Check sheet for the modelled part. Datum: model origin and axes. Units: mm. Face numbers are marked on the shaded views. A direction names the side the tool comes from. Coordinates: 2 decimals unless noted, no trailing zeros. Loops run counter-clockwise (first coordinate to the right, second up) from the corner with the lowest first, then second, coordinate; pieces in that order, holes last.
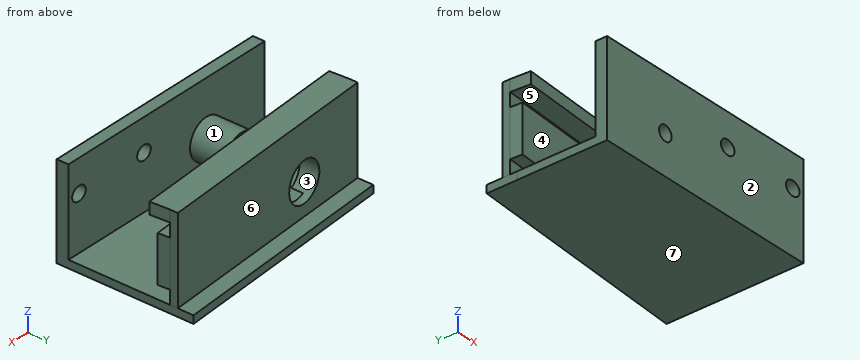
Autodesk Inventor part; units mm, degrees
ref_plane "YZ Plane" through (0, 0, 0) normal (1, 0, 0) x (0, 1, 0)
ref_plane "XZ Plane" through (0, 0, 0) normal (0, 1, 0) x (-1, 0, 0)
ref_plane "XY Plane" through (0, 0, 0) normal (0, 0, 1) x (1, 0, 0)
ref_plane "작업 평면1" through (-108.7402, -145.9081, -64.7043) normal (0, -1, 0) x (1, 0, 0)
sketch "스케치1" plane through (-108.7402, -145.9081, -64.7043) normal (0, -1, 0) x (1, 0, 0)
  ellipse E0 centre (-21.9712, -11.93) end of major axis (-19.8923, -11.93) minor radius 1.7957
  ellipse E1 centre (-2.1698, -11.93) end of major axis (-0.091, -11.93) minor radius 1.7957
  line L0 (-25.1804, -13.5798) -> (-25.1804, 0)
  ellipse E2 centre (0, 0) end of major axis (1.0394, 0) minor radius 0.8978 (1.0394, 0) -> (0, 0.8978) ccw
  line L1 (1.0394, 0) -> (1.0394, -13.5798)
  ellipse E3 centre (-0.2599, -13.5798) end of major axis (1.0394, -13.5798) minor radius 1.1223 (-0.2599, -14.7021) -> (1.0394, -13.5798) ccw
  line L2 (-0.2599, -14.7021) -> (-23.8811, -14.7021)
  ellipse E4 centre (-23.8811, -13.5798) end of major axis (-22.5818, -13.5798) minor radius 1.1223 (-25.1804, -13.5798) -> (-23.8811, -14.7021) ccw
  line L3 (-25.1804, -13.5798) -> (-25.1804, 0)
  ellipse E5 centre (-24.141, 0) end of major axis (-25.1804, 0) minor radius 0.8978 (-24.141, 0.8978) -> (-25.1804, 0) ccw
  line L4 (-24.141, 0.8978) -> (0, 0.8978)
  ellipse E6 centre (-21.9712, -11.93) end of major axis (-19.3726, -11.93) minor radius 2.2446
  ellipse E7 centre (-2.1698, -11.93) end of major axis (0.4288, -11.93) minor radius 2.2446
  ellipse E8 centre (-23.6213, -0.5275) end of major axis (-22.4194, -0.5275) minor radius 1.0381
  ellipse E9 centre (-20.3211, -0.5275) end of major axis (-19.1192, -0.5275) minor radius 1.0381
  ellipse E10 centre (-17.0208, -0.5275) end of major axis (-15.819, -0.5275) minor radius 1.0381
  ellipse E11 centre (-13.7206, -0.5275) end of major axis (-12.5188, -0.5275) minor radius 1.0381
  ellipse E12 centre (-10.4204, -0.5275) end of major axis (-9.2185, -0.5275) minor radius 1.0381
  ellipse E13 centre (-7.1202, -0.5275) end of major axis (-5.9183, -0.5275) minor radius 1.0381
  ellipse E14 centre (-3.8199, -0.5275) end of major axis (-2.6181, -0.5275) minor radius 1.0381
  ellipse E15 centre (-0.5197, -0.5275) end of major axis (0.6821, -0.5275) minor radius 1.0381
  line L5 (-25.1804, -3.7021) -> (1.0394, -3.7021)
  line L6 (1.0394, -27.7021) -> (-58.6804, -27.7021)
  line L7 (-58.6804, -27.7021) -> (-58.6804, -3.7021)
  line L8 (-58.6804, -3.7021) -> (1.0394, -3.7021)
  line L9 (1.0394, -3.7021) -> (1.0394, -27.7021)
  point P0 (108.7402, 64.7043)
  point P1 (-25.1804, -3.7021)
  point P2 (-25.1804, -3.7021)
  point P3 (1.0394, -13.5798)
  dimension "d0" = 11
  dimension "d3" = 33.5
  dimension "d4" = 13
extrude "돌출1" add sketch "스케치1" along normal blind 3 contours E4 L2 E3 L9 L6 L7 L8 L0 | L0 L5 L1 E3 L2 E4 | E6 | E7
sketch "스케치2" plane through (-108.7402, -145.9081, -64.7043) normal (0, 1, 0) x (1, 0, 0)
  line L0 (1.0394, 27.7021) -> (1.0394, 3.7021)
  line L1 (-58.6804, 27.7021) -> (1.0394, 27.7021)
  line L2 (-58.6804, 3.7021) -> (-58.6804, 27.7021)
  line L3 (1.0394, 27.7021) -> (-58.6804, 27.7021)
  line L4 (-58.6804, 27.7021) -> (-58.6804, 25.7021)
  line L5 (-58.6804, 25.7021) -> (1.0394, 25.7021)
  line L6 (1.0394, 25.7021) -> (1.0394, 27.7021)
  point P0 (108.7402, -64.7043)
  point P1 (1.0394, 25.7021)
  dimension "d5" = 2
extrude "돌출2" add sketch "스케치2" along normal blind 20
sketch "스케치4" plane through (-107.7008, -148.9081, -92.4064) normal (0, 0, -1) x (-1, 0, 0)
  line L0 (0, 23) -> (59.7199, 23)
  line L1 (0, 23) -> (0, 35)
  line L2 (0, 35) -> (42.7199, 35) construction
  line L3 (42.7199, 35) -> (42.7199, 32) construction
  line L4 (0, 35) -> (59.7199, 30.8062)
  line L5 (59.7199, 23) -> (59.7199, 40.663)
  point P0 (-107.7008, 148.9081)
  dimension "d11" = 42.7199
  dimension "d12" = 12
  dimension "d13" = 3
extrude "돌출4" add sketch "스케치4" against normal blind 2
sketch "스케치5" plane through (-108.7402, -145.9081, -64.7043) normal (0, 1, 0) x (1, 0, 0)
  line L0 (1.0394, 3.7021) -> (-58.6804, 3.7021)
  line L1 (1.0394, 25.7021) -> (1.0394, 3.7021)
  circle A0 centre (-40.9606, 17.7021) radius 5
  point P0 (108.7402, -64.7043)
  dimension "d16" = 10
  dimension "d17" = 14
  dimension "d18" = 42
extrude "돌출5" add sketch "스케치5" along normal blind 9
sketch "스케치6" plane through (-167.4206, -145.9081, -90.4064) normal (0, 0, 1) x (1, 0, 0)
  line L0 (59.7199, 0) -> (59.7199, 32)
  line L1 (59.7199, 32) -> (0, 27.8062)
  line L2 (0, 0) -> (0, 27.8062)
  line L3 (59.7199, 25.9852) -> (0, 21.7914)
  line L4 (59.7199, 27.9901) -> (0, 23.7963)
  line L5 (0, 23.7963) -> (0, 21.7914)
  line L6 (59.7199, 27.9901) -> (59.7199, 25.9852)
  point P0 (167.4206, 145.9081)
  point P1 (0, 23.7963)
  dimension "d21" = 6
  dimension "d22" = 2
extrude "돌출6" add sketch "스케치6" along normal up to surface (22 mm away) contours L3 L2 L4 L0
sketch "스케치11" plane through (-167.4206, -124.1167, -90.4064) normal (0.0701, -0.9975, 0) x (0.9975, 0.0701, 0)
  line L0 (59.8669, 22) -> (0, 22)
  line L1 (0, 0) -> (0, 22)
  line L2 (59.8669, 0) -> (0, 0)
  line L3 (59.8669, 0) -> (59.8669, 22)
  line L4 (0, 15.5) -> (59.8669, 15.5)
  line L5 (57.8365, 22) -> (-1.7367, 22)
  line L6 (0, 3.5) -> (59.8669, 3.5)
  point P0 (175.704, 90.4064)
  dimension "d36" = 6.5
  dimension "d39" = 3.5
extrude "돌출11" add sketch "스케치11" along normal blind 3 contours L3 L6 L1 L4
sketch "스케치7" plane through (-149.7008, -136.9081, -82.4064) normal (0, 1, 0) x (1, 0, 0)
  circle A0 centre (0, 0) radius 5
  circle A1 centre (0, 0) radius 1.9
  point P0 (149.7008, -82.4064)
  dimension "d25" = 3.8
extrude "돌출7" cut sketch "스케치7" against normal through all contours A1
sketch "스케치8" plane through (-149.7008, -136.9081, -82.4064) normal (0, 1, 0) x (1, 0, 0)
  circle A0 centre (0, 0) radius 5
  point P0 (149.7008, -82.4064)
extrude "돌출8" cut sketch "스케치8" along normal blind 16.75
sketch "스케치9" plane through (-167.4206, -124.1167, -90.4064) normal (0.0701, -0.9975, 0) x (0.9975, 0.0701, 0)
  line L0 (59.8669, 22) -> (0, 22)
  line L1 (0, 0) -> (0, 22)
  line L2 (59.8669, 0) -> (59.8669, 22)
  line L3 (0, 19) -> (59.8669, 19)
  point P0 (175.704, 90.4064)
  dimension "d30" = 3
extrude "돌출9" add sketch "스케치9" along normal blind 5
properties part number "IMU_base" material "고무, 검은색"
1) Set-up check for the marked faces 5, 6 and 7: record each of +Z, -Z, +X, -X, +Y, -Y from which the full face is reachable in a straight line by a thin tool's end or side.
Answer sheet:
face 5: +X
face 6: +Z, -X, +Y
face 7: -Z, +X, -X, +Y, -Y
2) Section check B-B on y = -143. Enter the section's corners in (x, z), plus the area to 3 significant figures.
Answer sheet:
outline: (-167.42, -92.41) - (-107.7, -92.41) - (-107.7, -90.41) - (-167.42, -90.41) - close; circle Ø10 at (-149.7, -82.41); hole circle Ø3.8 at (-149.7, -82.41)
area: 187 mm2
3) Scan lines: line 1 (Z direction, x = -157, y = -126); line 2 (Z direction, x = -135, y = -144); line 3 (Y direction, x = -119.5, z = -79). Record each from-to range of solid material in increasing order.
Answer sheet:
line 1: z = -92.41 to -90.41, -86.91 to -74.91, -71.41 to -68.41
line 2: z = -92.41 to -90.41
line 3: y = -148.91 to -145.91, -123.76 to -118.75
4) Mould release check, pull along X, two halves, no side actions. Record for the marked faces 1, 2, 3 and 4: +X half, -X half, draft (parallel to the pull), parting line (faces both ways), or undercut.
Answer sheet:
face 1: parting line
face 2: draft
face 3: undercut
face 4: +X half
5) Section check D-D on z = -89.25. Enter the section's corners in (x, y).
Answer sheet:
outline: (-167.42, -148.91) - (-107.7, -148.91) - (-107.7, -145.91) - (-167.42, -145.91) - close; (-167.42, -124.12) - (-107.7, -119.92) - (-107.7, -117.92) - (-167.42, -122.11) - close
6) Section check C-C on x = -151. Enter the section's corners in (y, z), plus the area to 3 significant figures.
Answer sheet:
outline: (-148.91, -92.41) - (-116.95, -92.41) - (-116.95, -90.41) - (-120.96, -90.41) - (-120.96, -87.23) - (-122.96, -87.23) - (-122.96, -90.41) - (-145.91, -90.41) - (-145.91, -87.23) - (-136.91, -87.23) - (-136.91, -83.79) - (-148.91, -83.79) - close; (-148.91, -81.02) - (-136.91, -81.02) - (-136.91, -77.58) - (-145.91, -77.58) - (-145.91, -68.41) - (-148.91, -68.41) - close; (-127.98, -71.41) - (-122.96, -71.41) - (-122.96, -74.91) - (-125.97, -74.91) - (-125.97, -77.58) - (-120.96, -77.58) - (-120.96, -68.41) - (-127.98, -68.41) - close
area: 231 mm2
7) Depth check by flat-ended pin: pin 1 (3 mm diameter, centred on x = -156.5, z = -87.5, fed in from +Y); pin 2 (5 mm diameter, centred on x = -149.7, z = -82.41, fed in from -Y); pin 3 (0.6 mm diameter, centred on y = -119.5, z = -77.5, fed in from +X); pin 4 (3 mm diameter, centred on x = -149, z = -80.5, fed in from +Y). Enter the tip coordinate at first touch or a pass-through.
Answer sheet:
pin 1: stops at y = -121.24
pin 2: stops at y = -148.91
pin 3: stops at x = -107.7
pin 4: stops at y = -136.91
